Check sheet for the modelled part. Datum: model origin and axes. Units: mm. A direction names the side the tool comes from. Coordinates: 2 decimals unless noted, no trailing zeros. Loops run counter-clockwise (first coordinate to the right, second up) from the corner with the lowest first, then second, coordinate; pieces in that order, holes last.
```python
from build123d import *

# Parameters (mm, degrees)
F0_R     = 20
F1_DEPTH = 15
F2_R     = 17.5
F3_DEPTH = 13
F4_R     = 3.5
F4_R_2   = 1.5
F5_DEPTH = 13


with BuildPart() as f1:
    # F0 (on Top) → F1 (new body)
    with BuildSketch(Plane.XY):
        Circle(F0_R)
    extrude(amount=F1_DEPTH)

    # F2 (on face) → F3 (cut)
    with BuildSketch(Plane.XY.offset(15)):
        Circle(F2_R)
    extrude(amount=-F3_DEPTH, mode=Mode.SUBTRACT)

    # F4 (on face) → F5 (join)
    with BuildSketch(Plane.XY.offset(2)):
        Circle(F4_R)
        Circle(F4_R_2, mode=Mode.SUBTRACT)
    extrude(amount=F5_DEPTH)


solid = f1.part
```
1) Mould release check, pull along X, two halves, no side actions. Record for faces 3 (the cylindrical face through (3.233, -1.341, 8.409)), 4 (the cylindrical face through (-4.336, -19.524, 7.395)), 5 (the flat face through (0, -18, 15)), 6 (the cylindrical face through (-1.5, 0.07, 8.41)): +X half, -X half, draft (parallel to the pull), parting line (faces both ways), or undercut.
Answer sheet:
face 3: undercut
face 4: parting line
face 5: draft
face 6: undercut
2) Set-up check for faces 1 (the flat face through (0, 0, 0)), 2 (the flat face through (0, -4, 2)): record each of +Z, -Z, +X, -X, +Y, -Y from which the full face is reachable in a straight line by a thin tool's end or side.
Answer sheet:
face 1: -Z, +X, -X, +Y, -Y
face 2: +Z
3) Section check A-A on x = 0. Enter the section's corners in (y, z), plus the area to 3 significant figures.
Answer sheet:
outline: (-20, 0) - (20, 0) - (20, 15) - (17.5, 15) - (17.5, 2) - (3.5, 2) - (3.5, 15) - (1.5, 15) - (1.5, 2) - (-1.5, 2) - (-1.5, 15) - (-3.5, 15) - (-3.5, 2) - (-17.5, 2) - (-17.5, 15) - (-20, 15) - close
area: 197 mm2
4) Scan lines: line 1 (Y direction, x = 0, z = 6.5); line 2 (Y direction, x = 2.5, z = 3.25); line 3 (Z direction, x = 8.5, y = 12). Record each from-to range of solid material in increasing order.
Answer sheet:
line 1: y = -20 to -17.5, -3.5 to -1.5, 1.5 to 3.5, 17.5 to 20
line 2: y = -19.84 to -17.32, -2.45 to 2.45, 17.32 to 19.84
line 3: z = 0 to 2
5) Section check D-D on x = 4. Enter the section's corners in (y, z).
Answer sheet:
outline: (-19.6, 0) - (19.6, 0) - (19.6, 15) - (17.04, 15) - (17.04, 2) - (-17.04, 2) - (-17.04, 15) - (-19.6, 15) - close
6) Depth check by flat-ended pin: pin 1 (6 mm diameter, centred on x = -9, y = 6, fed in from +Z); pin 2 (2 mm diameter, centred on y = -15, z = 7.5, fed in from +X); pin 3 (1 mm diameter, centred on y = -12, z = 3.5, fed in from +X). Enter the tip coordinate at first touch or a pass-through.
Answer sheet:
pin 1: stops at z = 2
pin 2: stops at x = 14.28
pin 3: stops at x = 16.36
7) Section check B-B on z = 10. Enter the section's corners in (x, y), plus the area to 3 significant figures.
Answer sheet:
outline: circle Ø40 at (0, 0); circle Ø7 at (0, 0); hole circle Ø35 at (0, 0); hole circle Ø3 at (0, 0)
area: 326 mm2
